Solid Edge part; units mm, degrees
sketch "Sketch1" plane through (0, 0, 0) normal (0, 0, 1) x (1, 0, 0)
  line L0 (4, -4) -> (4, 4)
  line L1 (4, 4) -> (-4, 4)
  line L2 (-4, 4) -> (-4, -4)
  line L3 (-4, -4) -> (4, -4)
extrude "ExtrudedProtrusion_1" add sketch "Sketch1" against normal blind 4
sketch "Sketch2" plane through (0, 0, 0) normal (0, 0, 1) x (0, 1, 0)
  circle A0 centre (0, 0) radius 3.5
extrude "ExtrudedCutout_1" cut sketch "Sketch2" against normal blind 1.2
fillet "Round_1" radius 1 4 edges at (4, -4, -2) (-4, -4, -2) (4, 4, -2) (-4, 4, -2)
sketch "Sketch3" plane through (0, 0, 0) normal (0, 0, 1) x (1, 0, 0)
  line L0 (4, -3) -> (4, 3)
  arc A0 (4, 3) -> (3, 4) centre (3, 3) ccw
  line L1 (3, 4) -> (-3, 4)
  arc A1 (-3, 4) -> (-4, 3) centre (-3, 3) ccw
  line L2 (-4, 3) -> (-4, -3)
  arc A2 (-4, -3) -> (-3, -4) centre (-3, -3) ccw
  line L3 (-3, -4) -> (3, -4)
  arc A3 (3, -4) -> (4, -3) centre (3, -3) ccw
  line L4 (4.5, -4.5) -> (4.5, 4.5)
  line L5 (4.5, 4.5) -> (-4.5, 4.5)
  line L6 (-4.5, 4.5) -> (-4.5, -4.5)
  line L7 (-4.5, -4.5) -> (4.5, -4.5)
extrude "ExtrudedProtrusion_2" add sketch "Sketch3" against normal blind 1
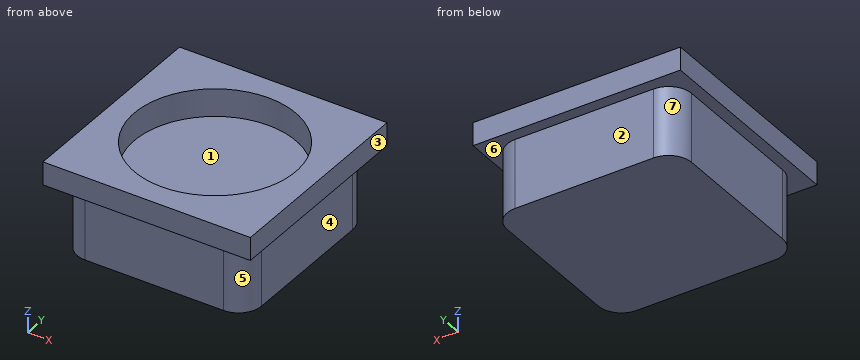
Can you work these out from the model? Positions are in its coordinate system, mm. Face numbers are marked on the shaded views. A direction names the side the tool comes from. Give positions to 0.01 mm unless a question says otherwise; leave off trailing zeros. Write each loop counter-clockwise with the first axis right and the second up, starting at its lowest first coordinate (ties: lowest second). Pieces come first, ordered by that corner, then holes. Notation, with made-up numbers: (13, -22.75) - (70, -22.75) arc R35 ccw to (70, 16.25) - close; hole circle Ø1 at (87, 26). An arc over 180 degrees is marked (long way). Write item = value, one per line. Start each with the question number.
1. Please list where these lines run through material, in increasing order: line 1 (Y direction, x = 0, z = -0.3); line 2 (Z direction, x = 2.75, y = -1).
2. Thinking about a two-plate mould opening in X: for the marked faces 1, 2 and 3, which applies, released by +X, released by -X, zero draft, split by the parting line, or undercut?
3. Imagine slicing it at A-A (z = -0.25). Please give me the cut outline in (x, y).
4. Imagine slicing it at D-D (z = -3.65). Please give me the cut outline in (x, y), and give its area (3 significant figures).
5. Imagine slicing it at B-B (y = 0). Please give me the cut outline in (x, z).
6. For pin 1 (1.5 mm diameter, centred on y = -1, z = -3, fed in from +X); pin 2 (0.9 mm diameter, centred on y = -1, z = -3, fed in from -X); pin 3 (1.5 mm diameter, centred on x = -0.5, z = -2, fed in from +Y), each with a flat end and sliding along its axis, tell me the tip position at first contact or that it passes through.
7. On a 3-axis mill with a long thin cutter (end or side, diameter ignored), from which of +Z, -Z, +X, -X, +Y, -Y can I reach the whole of each face in a straight line? I mean the marked faces 4, 5, 6 and 7. Say none if no direction works.
Worked answers:
q1.line_1 = -4.5 to -3.5, 3.5 to 4.5
q1.line_2 = -4 to -1.2
q2.face_1 = undercut
q2.face_2 = zero draft
q2.face_3 = released by +X
q3.outline = (-4.5, -4.5) - (4.5, -4.5) - (4.5, 4.5) - (-4.5, 4.5) - close; hole circle Ø7 at (0, 0)
q4.outline = (-4, -3) arc R1 ccw to (-3, -4) - (3, -4) arc R1 ccw to (4, -3) - (4, 3) arc R1 ccw to (3, 4) - (-3, 4) arc R1 ccw to (-4, 3) - close
q4.area = 63.1 mm2
q5.outline = (-4.5, -1) - (-4, -1) - (-4, -4) - (4, -4) - (4, -1) - (4.5, -1) - (4.5, 0) - (3.5, 0) - (3.5, -1.2) - (-3.5, -1.2) - (-3.5, 0) - (-4.5, 0) - close
q6.pin_1 = 4
q6.pin_2 = -4
q6.pin_3 = 4
q7.face_4 = -Z, +X, +Y, -Y
q7.face_5 = -Z, +X, -Y
q7.face_6 = -Z
q7.face_7 = -Z, -X, +Y
